```python
from build123d import *

# Parameters (mm, degrees)
F0_R     = 6.35
F1_DEPTH = 6.35
F2_R     = 6.34999


# Not quite as in the source:
# - a fillet or chamfer is up to 0.001 mm smaller than in the source, because OpenCascade refuses the exact size


with BuildPart() as f1:
    # F0 (on Top) → F1 (new body, symmetric)
    with BuildSketch(Plane.XY):
        with BuildLine():
            ThreePointArc((6.35, -15.4118372222), (0, 16.66875), (-6.35, -15.4118372222))
            Line((-6.35, -15.4118372222), (-6.35, -53.5118372222))
            Line((-6.35, -53.5118372222), (6.35, -53.5118372222))
            Line((6.35, -53.5118372222), (6.35, -15.4118372222))
        make_face()
        Circle(F0_R, mode=Mode.SUBTRACT)
    extrude(amount=F1_DEPTH, both=True)

    # F2 (radius 6.35 in the source; OpenCascade refuses exactly that, so slightly less here)
    f2_edges = [f1.edges().sort_by_distance(p)[0] for p in [
        (-6.35, -34.461837, -6.35),
        (6.35, -34.461837, -6.35),
        (-6.35, -34.461837, 6.35),
        (6.35, -34.461837, 6.35),
    ]]
    fillet(f2_edges, radius=F2_R)


solid = f1.part
```
Could you check a few things on this model? Use its own coordinates, in mm. A direction names the side the tool comes from. Coordinates: 2 decimals unless noted, no trailing zeros. Write each loop counter-clockwise with the first axis right and the second up, starting at its lowest first coordinate (ties: lowest second). Pieces come first, ordered by that corner, then holes. Notation, with made-up numbers: (56.5, 25.25) -> (79.5, 25.25) arc R23 cw to (79.5, 57.25) -> close; hole circle Ø9 at (38.5, -7). An arc over 180 degrees is marked (long way). Write item = value, one per line. Start each with the question number.
(1) I want a section at A-A (y = 0). Please give me the cut outline in (x, z), plus the area to 3 significant figures.
(2) I want a section at D-D (z = -2.5). Please give me the cut outline in (x, y), plus the area to 3 significant figures.
(3) I need wall thicknesses on line 1 (Y direction, x = 0, z = 2.75); line 2 (X direction, y = -35, z = 0.25); line 3 (X direction, y = 1, z = -0.25). Which ranges of each line are inside material? Lowest first, please. Write a range as [from, to].
(4) We'd pull the mould along X, two halves only. Please class faces 1 (the face through (-4.54, -34.73, -4.44)), 2 (the face through (0.733, 16.653, 0.089)), 3 (the face through (-1.38, -6.2, -0.09)): released by +X, released by -X, zero draft, split by the parting line, or undercut.
(5) Will these pins go through, and if not, where does the flat tip stop? pin 1 (1.5 mm diameter, centred on x = -5.5, y = -23, fed in from -Z); pin 2 (4 mm diameter, centred on x = -8.5, z = -4, fed in from +Y); pin 3 (3 mm diameter, centred on x = -6.5, y = -23.5, fed in from +Z).
(6) Which directions (+Z, -Z, +X, -X, +Y, -Y) give clear straight access to the entire face, cutting with the end or side of a thin tool? Please do faces 4 (the face through (-4.44, -34.73, 4.54)), 5 (the face through (4.54, -34.2, -4.44)), 6 (the face through (4.54, -34.2, 4.44)).
(7) I want a section at C-C (x = 1.5). Please give me the cut outline in (y, z).
Result set:
q1.outline = (-16.67, -6.35) -> (-6.35, -6.35) -> (-6.35, 6.35) -> (-16.67, 6.35) -> close; (6.35, -6.35) -> (16.67, -6.35) -> (16.67, 6.35) -> (6.35, 6.35) -> close
q1.area = 262 mm2
q2.outline = (-5.84, -53.51) -> (5.84, -53.51) -> (5.84, -15.61) arc R16.67 ccw (long way) to (-5.84, -15.61) -> close; hole circle Ø12.7 at (0, 0)
q2.area = 1,180 mm2
q3.line_1 = [-53.51, -6.35], [6.35, 16.67]
q3.line_2 = [-6.35, 6.35]
q3.line_3 = [-16.64, -6.27], [6.27, 16.64]
q4.face_1 = released by -X
q4.face_2 = split by the parting line
q4.face_3 = undercut
q5.pin_1 = -4.21
q5.pin_2 = 15.35
q5.pin_3 = 3.91
q6.face_4 = +Z, -X, -Y
q6.face_5 = -Z, +X, -Y
q6.face_6 = +Z, +X, -Y
q7.outline = (-53.51, -6.17) -> (-16.6, -6.17) -> (-16.6, -6.35) -> (-6.17, -6.35) -> (-6.17, 6.35) -> (-16.6, 6.35) -> (-16.6, 6.17) -> (-53.51, 6.17) -> close; (6.17, -6.35) -> (16.6, -6.35) -> (16.6, 6.35) -> (6.17, 6.35) -> close
